Build history of the part. All positions in model axes, mm. Face numbers are marked on the shaded views. A direction names the side the tool comes from. Give positions to 0.01 mm unless a question says otherwise; leave off trailing zeros. Order: outer loops, then holes, each group sorted by start corner. A loop starts at its lowest first (then second) coordinate and runs counter-clockwise, first axis right, second up. Notation, with made-up numbers: (-24, -33) - (4, -33) arc R3 ccw to (4, -29) - close; hole circle Ø9 at (44, 69). An arc over 180 degrees is marked (long way). Write each question's results on one line, items separated by ' | '. Start each with the question number.
Autodesk Inventor part; units mm, degrees
ref_plane "Work Plane1" through (-180, 0, 0) normal (-1, 0, 0) x (0, 0, 1)
ref_plane "YZ Plane" through (0, 0, 0) normal (1, 0, 0) x (0, 1, 0)
ref_plane "XZ Plane" through (0, 0, 0) normal (0, 1, 0) x (-1, 0, 0)
sketch "Sketch1" plane through (0, 0, 0) normal (1, 0, 0) x (0, 1, 0)
  circle A0 centre (0, 0) radius 19.85
  line L0 (-180, 0) -> (0, 0) construction
  line L1 (-180, 0) -> (-180, -60)
  arc A1 (4.753, -34.6758) -> (4.753, 34.6758) centre (0, 0) ccw
  line L2 (-180, -60) -> (4.753, -34.6758)
  line L3 (-180, 0) -> (-180, 60)
  line L4 (-180, 60) -> (4.753, 34.6758)
  dimension "d0" = 39.7
  dimension "d32" = 60
  dimension "d33" = 70
  dimension "d49" = 180
extrude "Extrusion1" add sketch "Sketch1" along normal blind 10
ref_plane "Work Plane1" through (-180, 0, 0) normal (-1, 0, 0) x (0, 0, 1)
sketch "Sketch2" plane through (-180, 0, 0) normal (-1, 0, 0) x (0, 0, 1)
  circle A0 centre (0, 0) radius 19.85
  line L0 (60, -180) -> (-60, -180)
  line L1 (34.6758, 4.753) -> (60, -180)
  arc A1 (34.6758, 4.753) -> (-34.6758, 4.753) centre (0, 0) ccw
  line L2 (-60, -180) -> (-34.6758, 4.753)
  circle A2 centre (0, 0) radius 19.85
extrude "Extrusion2" add sketch "Sketch2" along normal blind 10
sketch "Sketch5" plane through (0, -180, -50) normal (0, -1, 0) x (1, 0, 0)
  arc A0 (60, 50) -> (-240, 50) centre (-90, 50) ccw
  line L0 (-90, 50) -> (35, 50) construction
  circle A1 centre (25.7561, 54.9891) radius 1.5
  circle A2 centre (35.3012, 39.5) radius 1.5
  circle A3 centre (43.9427, 55.5109) radius 1.5
  circle A4 centre (35, 50) radius 13.5 construction
  circle A5 centre (-215.3012, 39.5) radius 1.5
  circle A6 centre (-205.7561, 54.9891) radius 1.5
  circle A7 centre (-215, 50) radius 13.5 construction
  circle A8 centre (-223.9427, 55.5109) radius 1.5
  line L1 (60, 50) -> (-240, 50)
  line L2 (-240, 50) -> (-240, -100)
  line L3 (-240, -100) -> (60, -100)
  line L4 (60, -100) -> (60, 50)
  circle A9 centre (-90, 50) radius 10
  line L5 (-180, -10) -> (-180, 110) construction
  line L6 (-180, 50) -> (0, 50) construction
  line L7 (0, 110) -> (0, -10) construction
  line L8 (-90, 50) -> (-90, 90)
  line L9 (-215, 50) -> (-152.5, 158.2532) construction
  line L10 (-152.5, 158.2532) -> (-27.5, 158.2532) construction
  line L11 (-27.5, 158.2532) -> (35, 50) construction
  line L12 (35, 50) -> (-27.5, -58.2532) construction
  line L13 (-27.5, -58.2532) -> (-152.5, -58.2532) construction
  line L14 (-152.5, -58.2532) -> (-215, 50) construction
  circle A10 centre (-152.1988, -68.7532) radius 1.5
  circle A11 centre (-161.7439, -53.264) radius 1.5
  circle A12 centre (-152.5, -58.2532) radius 13.5 construction
  circle A13 centre (-143.5573, -52.7423) radius 1.5
  circle A14 centre (-27.1988, -68.7532) radius 1.5
  circle A15 centre (-36.7439, -53.264) radius 1.5
  circle A16 centre (-27.5, -58.2532) radius 13.5 construction
  circle A17 centre (-18.5573, -52.7423) radius 1.5
  circle A18 centre (-152.1988, 147.7532) radius 1.5
  circle A19 centre (-161.7439, 163.2423) radius 1.5
  circle A20 centre (-152.5, 158.2532) radius 13.5 construction
  circle A21 centre (-143.5573, 163.764) radius 1.5
  circle A22 centre (-27.1988, 147.7532) radius 1.5
  circle A23 centre (-36.7439, 163.2423) radius 1.5
  circle A24 centre (-27.5, 158.2532) radius 13.5 construction
  circle A25 centre (-18.5573, 163.764) radius 1.5
  line L15 (-65, 75) -> (-115, 75) construction
  line L16 (-115, 75) -> (-115, 25) construction
  line L17 (-115, 25) -> (-65, 25) construction
  line L18 (-65, 25) -> (-65, 75) construction
  line L19 (-65, 75) -> (-115, 25) construction
  line L20 (-115, 75) -> (-65, 25) construction
  circle A26 centre (-65, 75) radius 2.5
  circle A27 centre (-115, 75) radius 2.5
  circle A28 centre (-65, 25) radius 2.5
  circle A29 centre (-115, 25) radius 2.5
  point P0 (35, 50)
  point P1 (35, 50)
  point P2 (35, 50)
  point P3 (-215, 50)
  point P4 (-215, 50)
  point P5 (-215, 50)
  point P6 (-215, 50)
  point P7 (-152.5, -58.2532)
  point P8 (-152.5, -58.2532)
  point P9 (-152.5, -58.2532)
  point P10 (-152.5, -58.2532)
  point P11 (-27.5, -58.2532)
  point P12 (-27.5, -58.2532)
  point P13 (-27.5, -58.2532)
  point P14 (-27.5, -58.2532)
  point P15 (-152.5, 158.2532)
  point P16 (-152.5, 158.2532)
  point P17 (-152.5, 158.2532)
  point P18 (-152.5, 158.2532)
  point P19 (-27.5, 158.2532)
  point P20 (-27.5, 158.2532)
  point P21 (-27.5, 158.2532)
  point P22 (-27.5, 158.2532)
  point P23 (-90, 50)
  dimension "d21" = 300
  dimension "d25" = 125
  dimension "d30" = 20
  dimension "d34" = 40
  dimension "d35" = 150
  dimension "d36" = 50
  dimension "d37" = 50
  dimension "d38" = 5
extrude "Extrusion5" add sketch "Sketch5" along normal blind 10 contours L1 A9 A0 | L4 L3 L2 L1 A9
fillet "Fillet1" radius 30 2 edges at (-240, -185, -150) (60, -185, -150)
sketch "Sketch8" plane through (60, -190, 0) normal (1, 0, 0) x (0, 0, -1)
  line L0 (60, 10) -> (-60, 10)
  line L1 (60, 10) -> (105, 10)
  line L2 (0, 10) -> (120, 10)
  line L3 (105, 10) -> (105, 31) construction
  circle A0 centre (105, 31) radius 8.5527
  point P0 (0, 190)
  dimension "d44" = 45
  dimension "d45" = 21
extrude "Extrusion7" [suppressed]
properties part number "Foundation-Fork"
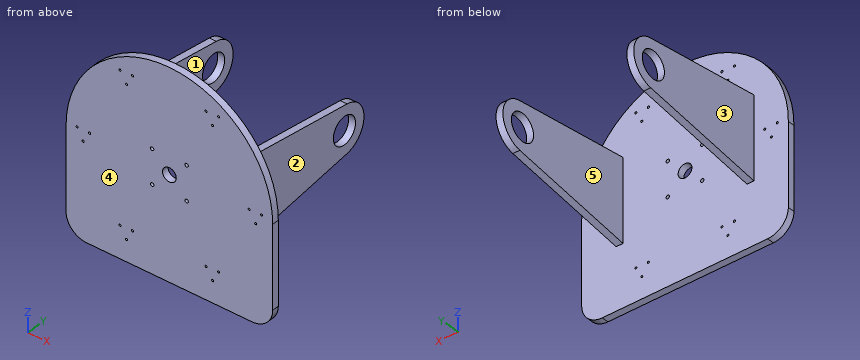
Item 1: Flat gauge pins, fed straight in: pin 1 Ø10 at (x, z) = (7, 14) entering from +Y; pin 2 Ø6.5 at (x, z) = (-115, 25) entering from +Y; pin 3 Ø2 at (x, y) = (-183, -85.5) entering from -Z. Where does each tip first touch, or does it go through?
Item 2: Cut at C-C, the plane x = -125.5. List the corners of the cut face in (y, z).
Item 3: Cut at B-B, the plane y = 0. List the corners of the cut face in (x, z).
Item 4: Two-plate mould, pull along X, no slides. Class the marked faces 3, 4 and 5: +X half, -X half, draft (parallel to the pull), parting line (faces both ways), or undercut.
Item 5: Cut at A-A, the plane y = -131. List the corners of the cut face in (x, z).
Item 6: Which spindle directions (+Z, -Z, +X, -X, +Y, -Y) get a long thin tool onto all of the face, cutting with end or side? Do the marked faces 1 and 2. Say none if no direction does.
Item 7: Probe line 1 along X through (y, z) = (-174.5, 54); line 2 along Z through (x, y) = (-90, -182.5); line 3 along Y through (x, z) = (-157, -136). List the from-to ranges inside material, lowest first. Write a range as from..to.
Item 8: Cut at D-D, the plane z = -85. List the corners of the cut face in (x, y), then the cut area to 3 significant figures.
Values found:
1) pin 1: stops at y = 33.82 | pin 2: stops at y = -180 | pin 3: stops at z = -47.18
2) outline: (-190, -150) - (-180, -150) - (-180, 145.74) - (-190, 145.74) - close
3) outline: (-190, -35.33) - (-180, -35.33) - (-180, -19.85) - (-190, -19.85) - close; (-190, 19.85) - (-180, 19.85) - (-180, 35.33) - (-190, 35.33) - close; (0, -35.33) - (10, -35.33) - (10, -19.85) - (0, -19.85) - close; (0, 19.85) - (10, 19.85) - (10, 35.33) - (0, 35.33) - close
4) face 3: -X half | face 4: draft | face 5: undercut
5) outline: (-190, -53.28) - (-180, -53.28) - (-180, 53.28) - (-190, 53.28) - close; (0, -53.28) - (10, -53.28) - (10, 53.28) - (0, 53.28) - close
6) face 1: +Z, -Z, +Y | face 2: +Z, -Z, +X, +Y
7) line 1: x = -190..-180, 0..10 | line 2: z = -150..-10, 10..150 | line 3: y = -190..-180
8) outline: (-240, -190) - (60, -190) - (60, -180) - (-240, -180) - close | area: 3,000 mm2
